```python
from build123d import *

# Parameters (mm, degrees)
F0_W     = 67.3768445849
F0_H     = 98.9107750356
F0_W_2   = 2.7784528211
F0_H_2   = 29.5537686782
F0_H_3   = 2.1962313218
F0_H_4   = 28.8333376633
F0_W_3   = 28.9715471789
F0_W_4   = 31.75
F0_H_5   = 2.9166623367
F0_H_6   = 31.75
F1_DEPTH = 19.558
F2_DEPTH = 3.302


with BuildPart() as f1:
    # F0 (on Top) → F1 (new body)
    with BuildSketch(Plane.XY):
        with Locations((-0.175267458, 3.9172600955)):
            Rectangle(F0_W, F0_H)
        Polygon((-31.75, 22.0649391413), (-31.75, 51.6187078194), (-2.7784528211, 51.6187078194), (0, 51.6187078194), (31.75, 51.6187078194), (31.75, 22.0649391413), (31.75, 19.8687078194), (31.75, -8.9646298438), (31.75, -11.8812921806), (31.75, -43.6312921806), (0, -43.6312921806), (-2.7784528211, -43.6312921806), (-31.75, -43.6312921806), (-31.75, -11.8812921806), (-31.75, -8.9646298438), (-31.75, 19.8687078194), align=None, mode=Mode.SUBTRACT)
        with Locations((-1.3892264105, 36.8418234804)):
            Rectangle(F0_W_2, F0_H_2)
        with Locations((-1.3892264105, 20.9668234804)):
            Rectangle(F0_W_2, F0_H_3)
        with Locations((-1.3892264105, 5.4520389878)):
            Rectangle(F0_W_2, F0_H_4)
        with Locations((-17.2642264105, 20.9668234804)):
            Rectangle(F0_W_3, F0_H_3)
        with Locations((15.875, 20.9668234804)):
            Rectangle(F0_W_4, F0_H_3)
        with Locations((-17.2642264105, -10.4229610122)):
            Rectangle(F0_W_3, F0_H_5)
        with Locations((-1.3892264105, -10.4229610122)):
            Rectangle(F0_W_2, F0_H_5)
        with Locations((-1.3892264105, -27.7562921806)):
            Rectangle(F0_W_2, F0_H_6)
        with Locations((15.875, -10.4229610122)):
            Rectangle(F0_W_4, F0_H_5)
    extrude(amount=F1_DEPTH)

    # F0 (on Top) → F2 (join)
    with BuildSketch(Plane.XY):
        with Locations((-0.175267458, 3.9172600955)):
            Rectangle(F0_W, F0_H)
        Polygon((-31.75, 22.0649391413), (-31.75, 51.6187078194), (-2.7784528211, 51.6187078194), (0, 51.6187078194), (31.75, 51.6187078194), (31.75, 22.0649391413), (31.75, 19.8687078194), (31.75, -8.9646298438), (31.75, -11.8812921806), (31.75, -43.6312921806), (0, -43.6312921806), (-2.7784528211, -43.6312921806), (-31.75, -43.6312921806), (-31.75, -11.8812921806), (-31.75, -8.9646298438), (-31.75, 19.8687078194), align=None, mode=Mode.SUBTRACT)
        with Locations((15.875, 36.8418234804)):
            Rectangle(F0_W_4, F0_H_2)
        with Locations((15.875, 5.4520389878)):
            Rectangle(F0_W_4, F0_H_4)
        with Locations((-17.2642264105, 36.8418234804)):
            Rectangle(F0_W_3, F0_H_2)
        with Locations((-17.2642264105, 5.4520389878)):
            Rectangle(F0_W_3, F0_H_4)
        with Locations((-17.2642264105, -27.7562921806)):
            Rectangle(F0_W_3, F0_H_6)
        with Locations((15.875, -27.7562921806)):
            Rectangle(F0_W_4, F0_H_6)
    extrude(amount=F2_DEPTH)


solid = f1.part
```
For this review, take the finished solid that the model builds, in its own axes (mm). Coordinates: 2 decimals unless noted, no trailing zeros. Order: outer loops, then holes, each group sorted by start corner. A loop starts at its lowest first (then second) coordinate and runs counter-clockwise, first axis right, second up. Notation, with made-up numbers: (88, -36.5) - (113, -36.5) arc R10 cw to (113, -19.5) - close; hole circle Ø10 at (-31, -14). An arc over 180 degrees is marked (long way). Answer as a JSON object with one key per item and string values. Group by question number.
1. For probe 1 along Y at (x, z) = (-9, 8.5); probe 2 along X at (y, z) = (48, 16); probe 3 along Z at (x, y) = (-19.5, 40), list the stretches that pass through material, from the lowest coordinate up.
2. We need section C-C on y = 17. State the section outline as (x, z) points, then the cut area to 3 significant figures.
3. The part is to be moulded in two halves that separate along X. For faces 1 (the flat face through (-33.864, 3, 10)), 2 (the flat face through (-17, -11.881, 11)), 3 (the flat face through (16, -8.965, 11)), 4 (the flat face through (-1, 53.373, 10)), say which applies: pulls with the +X half, pulls with the -X half, needs draft (parallel to the pull), parting line crosses it, or undercut.
4. We need section A-A on z = 5.5. State the section outline as (x, y) points.
5. Clearance check with a flat-ended pin moving along its axis: P1, Ø14.5, axis at x = -10.5, y = 34.5, coming from the +Z side. State where the tip first meets the part, or that it passes through.
6. We need section B-B on x = -23.5. State the section outline as (y, z) points.
Final values:
{
 "1": {"probe 1": "-45.54 to -43.63, -11.88 to -8.96, 19.87 to 22.06, 51.62 to 53.37", "probe 2": "-33.86 to -31.75, -2.78 to 0, 31.75 to 33.51", "probe 3": "0 to 3.3"},
 "2": {"outline": "(-33.86, 0) - (33.51, 0) - (33.51, 19.56) - (31.75, 19.56) - (31.75, 3.3) - (0, 3.3) - (0, 19.56) - (-2.78, 19.56) - (-2.78, 3.3) - (-31.75, 3.3) - (-31.75, 19.56) - (-33.86, 19.56) - close", "area": "331 mm²"},
 "3": {"face 1": "pulls with the -X half", "face 2": "undercut", "face 3": "undercut", "face 4": "needs draft"},
 "4": {"outline": "(-33.86, -45.54) - (33.51, -45.54) - (33.51, 53.37) - (-33.86, 53.37) - close; hole (-31.75, -43.63) - (-2.78, -43.63) - (-2.78, -11.88) - (-31.75, -11.88) - close; hole (-31.75, -8.96) - (-2.78, -8.96) - (-2.78, 19.87) - (-31.75, 19.87) - close; hole (-31.75, 22.06) - (-2.78, 22.06) - (-2.78, 51.62) - (-31.75, 51.62) - close; hole (0, -43.63) - (31.75, -43.63) - (31.75, -11.88) - (0, -11.88) - close; hole (0, -8.96) - (31.75, -8.96) - (31.75, 19.87) - (0, 19.87) - close; hole (0, 22.06) - (31.75, 22.06) - (31.75, 51.62) - (0, 51.62) - close"},
 "5": {"P1": "z = 3.3"},
 "6": {"outline": "(-45.54, 0) - (53.37, 0) - (53.37, 19.56) - (51.62, 19.56) - (51.62, 3.3) - (22.06, 3.3) - (22.06, 19.56) - (19.87, 19.56) - (19.87, 3.3) - (-8.96, 3.3) - (-8.96, 19.56) - (-11.88, 19.56) - (-11.88, 3.3) - (-43.63, 3.3) - (-43.63, 19.56) - (-45.54, 19.56) - close"}
}
